```python
from build123d import *

# Parameters (mm, degrees)
BOSS_EXTRUDE1_DEPTH = 5.842
FILLET1_R           = 12.7
FILLET2_R           = 3.175
SKETCH2_R           = 0.1984375
CUT_EXTRUDE1_DEPTH  = 136.775443647


with BuildPart() as part:
    # Sketch1 → Boss-Extrude1 (new body)
    with BuildSketch(Plane.XY):
        with BuildLine():
            Line((-12.8, -25.5), (-6.35, -25.5))
            Line((-6.35, -25.5), (-6.35, -31.342))
            Line((-6.35, -31.342), (6.35, -31.342))
            Line((6.35, -31.342), (6.35, -25.5))
            Line((6.35, -25.5), (12.8, -25.5))
            Line((12.8, -25.5), (12.8, -19.05))
            Line((12.8, -19.05), (18.642, -19.05))
            Line((18.642, -19.05), (18.642, -6.35))
            Line((18.642, -6.35), (12.8, -6.35))
            Line((12.8, -6.35), (12.8, 6.35))
            Line((12.8, 6.35), (18.642, 6.35))
            Line((18.642, 6.35), (18.642, 19.05))
            Line((18.642, 19.05), (12.8, 19.05))
            Line((12.8, 19.05), (12.8, 25.5))
            Line((12.8, 25.5), (6.35, 25.5))
            Line((6.35, 25.5), (6.35, 31.342))
            Line((6.35, 31.342), (-6.35, 31.342))
            Line((-6.35, 31.342), (-6.35, 25.5))
            Line((-6.35, 25.5), (-12.8, 25.5))
            Line((-12.8, 25.5), (-12.8, 44.55))
            Line((-12.8, 44.55), (12.6, 44.55))
            ThreePointArc((12.6, 44.55), (21.721677477, 40.771677477), (25.5, 31.65))
            Line((25.5, 31.65), (25.5, 25.3))
            Line((25.5, 25.3), (25.5, -25.5))
            Line((25.5, -25.5), (12.7, -114.4))
            Line((12.7, -114.4), (0, -127.1))
            Line((0, -127.1), (-50.9, -114.4))
            Line((-50.9, -114.4), (-50.9, -101.7))
            Line((-50.9, -101.7), (-12.8, -101.7))
            Line((-12.8, -101.7), (-12.8, -25.5))
        make_face()
    extrude(amount=BOSS_EXTRUDE1_DEPTH)

    # Fillet1
    fillet1_edges = [part.edges().sort_by_distance(p)[0] for p in [
        (25.5, -25.5, 2.921),
        (12.7, -114.4, 2.921),
        (0, -127.1, 2.921),
        (-50.9, -114.4, 2.921),
    ]]
    fillet(fillet1_edges, radius=FILLET1_R)

    # Fillet2
    fillet2_edges = [part.edges().sort_by_distance(p)[0] for p in [
        (-12.8, 44.55, 2.921),
    ]]
    fillet(fillet2_edges, radius=FILLET2_R)

    # Sketch2 → Cut-Extrude1 (cut, through all)
    with BuildSketch(Plane.XY.offset(5.842)):
        with Locations((-6.35, 31.342)):
            Circle(SKETCH2_R)
        with Locations((6.35, 31.342)):
            Circle(SKETCH2_R)
        with Locations((18.642, 19.05)):
            Circle(SKETCH2_R)
        with Locations((12.8, 25.5)):
            Circle(SKETCH2_R)
        with Locations((18.642, 6.35)):
            Circle(SKETCH2_R)
        with Locations((18.642, -6.35)):
            Circle(SKETCH2_R)
        with Locations((12.8, -25.5)):
            Circle(SKETCH2_R)
        with Locations((18.642, -19.05)):
            Circle(SKETCH2_R)
        with Locations((6.35, -31.342)):
            Circle(SKETCH2_R)
        with Locations((-6.35, -31.342)):
            Circle(SKETCH2_R)
    extrude(amount=-CUT_EXTRUDE1_DEPTH, mode=Mode.SUBTRACT)


solid = part.part
```
CAD build for the part. Positions are in the model's coordinates, mm. A direction names the side the tool comes from. Coordinates: 2 decimals unless noted, no trailing zeros. Loops run counter-clockwise (first coordinate to the right, second up) from the corner with the lowest first, then second, coordinate; pieces in that order, holes last. Notation, with made-up numbers: (-21.5, 74) - (2.5, 74) arc R21 cw to (2.5, 91) - close; hole circle Ø1 at (79, 78). An arc over 180 degrees is marked (long way). Use CSV: the item, a comma, the result in double quotes. Start each with the question number.
Q1. Drop flat-ended pins along their axis: P1, Ø3, axis at x = -23.5, z = 4, coming from the -Y side; P2, Ø1, axis at y = -34.5, z = 1.5, coming from the -X side. Give the stop position or say it passes through.
Q2. Cut at B-B, the plane y = -40.5. List the corners of the cut face in (x, z).
Q3. Cut at C-C, the plane x = -22. List the corners of the cut face in (y, z).
Q4. 3-axis set-ups, long thin cutter, end or side, ignore diameter. For faces 1 (the cylindrical face through (21.62, 40.87, 2.88)), 2 (the flat face through (0, 31.342, 3)), 3 (the flat face through (12.8, -22, 3)), 4 (the flat face through (-32, -101.7, 3)): which of +Z, -Z, +X, -X, +Y, -Y reach the whole face in a straight line?
Q5. Cut at A-A, the plane x = 1.5. List the corners of the cut face in (y, z), then the cut area to 3 significant figures.
Q6. Two-plate mould, pull along Y, no slides. Class faces 5 (the flat face through (16, -6.35, 3)), 6 (the cylindrical face through (-0.417, -125.252, 2.962)), 7 (the flat face through (9, -25.5, 3)), 8 (the flat face through (-12.8, 33, 3)): +Y half, -Y half, draft (parallel to the pull), parting line (faces both ways), or undercut.
Q7. Probe probe 1 along X at (y, z) = (29, 2.3); probe 2 along X at (y, z) = (-73, 2.05); probe 3 along Y at (x, z) = (-2.5, 4.85). List the from-to ranges inside material, lowest first. Write a range as from..to.
Here are the results:
1,P1,"y = -121.61"
1,P2,"x = -12.8"
2,outline,"(-12.8, 0) - (23.34, 0) - (23.34, 5.84) - (-12.8, 5.84) - close"
3,outline,"(-121.61, 0) - (-101.7, 0) - (-101.7, 5.84) - (-121.61, 5.84) - close"
4,face 1,"+Z, -Z, +X, +Y"
4,face 2,"+Z, -Z"
4,face 3,"+Z, -Z, -X"
4,face 4,"+Z, -Z, -X, +Y"
5,outline,"(-124.53, 0) - (-31.34, 0) - (-31.34, 5.84) - (-124.53, 5.84) - close; (31.34, 0) - (44.55, 0) - (44.55, 5.84) - (31.34, 5.84) - close"
5,area,"622 mm2"
6,face 5,"undercut"
6,face 6,"-Y half"
6,face 7,"undercut"
6,face 8,"draft"
7,probe 1,"-12.8..-6.35, 6.35..25.5"
7,probe 2,"-12.8..18.66"
7,probe 3,"-125.66..-31.34, 31.34..44.55"
